Autodesk Fusion 360 part; units mm, degrees
sketch "Sketch2" plane through (0, 0, 0) normal (1, 0, 0) x (0, 0, -1)
  line L0 (0, 0) -> (0, 10)
  dimension "d53" = 10
sketch "Sketch1" plane through (0, 0, 0) normal (0, 1, 0) x (1, 0, 0)
  line L0 (0, 0) -> (141.9, 0)
  line L1 (141.9, 0) -> (141.9, 151.05)
  line L2 (0, 151.05) -> (0, 0)
  line L3 (130.925, 43.6) -> (10.975, 43.6) construction
  circle A0 centre (10.975, 43.6) radius 1.75
  circle A1 centre (130.925, 43.6) radius 1.75
  line L4 (70.95, 0) -> (70.95, 43.6) construction
  line L5 (65.95, 0) -> (68.5, 0)
  line L6 (70.95, -2) -> (65.95, -2)
  line L7 (65.95, -2) -> (65.95, 0)
  line L8 (75.95, -2) -> (75.95, 0)
  line L9 (70.95, -2) -> (75.95, -2)
  line L10 (70.95, 43.6) -> (70.95, 85.6) construction
  line L11 (72.7, 88.1) -> (72.7, 83.1)
  line L12 (69.2, 83.1) -> (69.2, 88.1)
  arc A2 (72.7, 88.1) -> (69.2, 88.1) centre (70.95, 88.1) ccw
  arc A3 (69.2, 83.1) -> (72.7, 83.1) centre (70.95, 83.1) ccw
  line L13 (69.2, 85.6) -> (72.7, 85.6) construction
  line L14 (3.35, 120.45) -> (44.05, 120.45) construction
  circle A4 centre (3.35, 120.45) radius 1.75
  circle A5 centre (44.05, 120.45) radius 1.75
  line L15 (23.7, 151.05) -> (23.7, 120.45) construction
  line L16 (7.7, 149.45) -> (39.7, 149.45)
  line L17 (39.7, 149.45) -> (39.7, 91.45)
  line L18 (39.7, 91.45) -> (7.7, 91.45)
  line L19 (7.7, 91.45) -> (7.7, 149.45)
  line L20 (134.2, 91.45) -> (134.2, 149.45)
  line L21 (134.2, 149.45) -> (102.2, 149.45)
  line L22 (102.2, 149.45) -> (102.2, 91.45)
  circle A6 centre (138.55, 120.45) radius 1.75
  line L23 (102.2, 91.45) -> (134.2, 91.45)
  circle A7 centre (97.85, 120.45) radius 1.75
  line L24 (48.95, 135.45) -> (92.95, 135.45)
  line L25 (92.95, 135.45) -> (92.95, 91.45)
  line L26 (92.95, 91.45) -> (48.95, 91.45)
  line L27 (48.95, 91.45) -> (48.95, 135.45)
  line L28 (48.95, 113.45) -> (39.7, 113.45) construction
  line L29 (92.95, 113.45) -> (102.2, 113.45) construction
  circle A8 centre (52.7, 131.7) radius 1.75
  circle A9 centre (52.7, 95.2) radius 1.75
  circle A10 centre (89.2, 95.2) radius 1.75
  circle A11 centre (89.2, 131.7) radius 1.75
  line L30 (74.1, 142.05) -> (74.1, 137.05)
  line L31 (74.1, 173.25) -> (74.1, 168.25)
  line L32 (82.45, 143.65) -> (82.45, 166.65)
  line L33 (74.1, 173.25) -> (79.95, 173.25)
  line L34 (57.85, 142.05) -> (74.1, 142.05)
  line L35 (74.1, 168.25) -> (57.85, 168.25)
  line L36 (57.85, 142.05) -> (57.85, 168.25)
  line L37 (78.35, 138.65) -> (78.35, 143.65)
  line L38 (78.35, 166.65) -> (78.35, 171.65)
  line L39 (82.45, 166.65) -> (78.35, 166.65)
  line L40 (78.35, 143.65) -> (82.45, 143.65)
  line L41 (75.7, 166.65) -> (59.45, 166.65)
  line L42 (59.45, 166.65) -> (59.45, 143.65)
  line L43 (75.7, 171.65) -> (75.7, 166.65)
  line L44 (59.45, 143.65) -> (75.7, 143.65)
  line L45 (78.35, 171.65) -> (75.7, 171.65)
  line L46 (75.7, 138.65) -> (78.35, 138.65)
  line L47 (75.7, 143.65) -> (75.7, 138.65)
  line L48 (84.05, 142.05) -> (79.95, 142.05)
  line L49 (79.95, 137.05) -> (74.1, 137.05)
  line L50 (84.05, 168.25) -> (84.05, 142.05)
  line L51 (79.95, 142.05) -> (79.95, 137.05)
  line L52 (79.95, 168.25) -> (79.95, 173.25)
  line L53 (84.05, 168.25) -> (79.95, 168.25)
  line L54 (82.45, 155.15) -> (59.45, 155.15) construction
  line L55 (70.95, 155.15) -> (70.95, 135.45) construction
  line L56 (56.25, 151.05) -> (56.25, 174.85)
  line L57 (56.25, 174.85) -> (85.65, 174.85)
  line L58 (85.65, 174.85) -> (85.65, 151.05)
  line L59 (141.9, 151.05) -> (85.65, 151.05)
  line L60 (56.25, 151.05) -> (0, 151.05)
  line L61 (59.45, 143.65) -> (57.85, 143.65)
  line L62 (59.45, 147.65) -> (57.85, 147.65)
  line L63 (74.1, 173.25) -> (57.85, 173.25)
  line L64 (57.85, 173.25) -> (57.85, 168.25)
  line L65 (79.95, 173.25) -> (84.05, 173.25)
  line L66 (84.05, 173.25) -> (84.05, 168.25)
  line L67 (75.95, -2) -> (75.95, -3.6)
  line L68 (75.95, -3.6) -> (65.95, -3.6)
  line L69 (65.95, -3.6) -> (65.95, -2)
  point P0 (70.95, 113.45)
  point P1 (-289, 70)
  dimension "d1" = 141.9
  dimension "d2" = 151.05
  dimension "d3" = 119.95
  dimension "d4" = 3.5
  dimension "d6" = 5
  dimension "d8" = 43.6
  dimension "d9" = 42
  dimension "d10" = 3.5
  dimension "d11" = 5
  dimension "d12" = 40.7
  dimension "d13" = 3.5
  dimension "d14" = 3.35
  dimension "d15" = 30.6
  dimension "d16" = 58
  dimension "d17" = 1.6
  dimension "d18" = 32
  dimension "d19" = 16
  dimension "d20" = 44
  dimension "d23" = 44
  dimension "d24" = 3.35
  dimension "d25" = 3.5
  dimension "d26" = 3.75
  dimension "d27" = 3.75
  dimension "d28" = 22
  dimension "d29" = 22
  dimension "d31" = 360
  dimension "d32" = 4.9
  dimension "d33" = 4.9
  dimension "d34" = 1.6
  dimension "d35" = 1.6
  dimension "d36" = 1.6
  dimension "d37" = 1.6
  dimension "d38" = 1.6
  dimension "d39" = 1.6
  dimension "d40" = 1.6
  dimension "d41" = 1.6
  dimension "d42" = 1.6
  dimension "d43" = 1.6
  dimension "d44" = 1.6
  dimension "d45" = 1.6
  dimension "d47" = 5
  dimension "d48" = 23
  dimension "d49" = 23
  dimension "d50" = 4.1
  dimension "d51" = 6.75
  dimension "d54" = 1.6
  dimension "d55" = 1.6
  dimension "d56" = 1.6
  dimension "d57" = 1.6
  dimension "d58" = 4
  dimension "d80" = 2
  dimension "d81" = 1.6
extrude "Extrude1" add sketch "Sketch1" against normal blind 4 contours L0 L1 L2 L5 L56 L57 L58 L59 L60 | L0 L5 L6 L7 L8 L9 | L6 L9 L67 L68 L69 | L16 L17 L18 L19 | L20 L21 L22 L23 | L24 L25 L26 L27 | L30 L31 L32 L33 L34 L35 L36 L37 L38 L39 L40 L41 L42 L43 L44 L45 L46 L47 L48 L49 L50 L51 L52 L53 L61 L62 | L36 L42 L61 L62 | L32 L37 L38 L39 L40 L41 L42 L43 L44 L45 L46 L47 | L31 L35 L63 L64 | L52 L53 L65 L66
extrude "Extrude2" cut sketch "Sketch1" against normal blind 1.6 contours L16 L17 L18 L19 | L20 L21 L22 L23 | L24 L25 L26 L27
extrude "Extrude3" add sketch "Sketch1" along normal blind 5 contours L6 L9 L67 L68 L69
extrude "Extrude4" add sketch "Sketch1" along normal blind 40 contours L30 L31 L32 L33 L34 L35 L36 L37 L38 L39 L40 L41 L42 L43 L44 L45 L46 L47 L48 L49 L50 L51 L52 L53 L61 L62 | L31 L35 L63 L64 | L52 L53 L65 L66
sketch "Sketch3" plane through (84.05, 0, 0) normal (1, 0, 0) x (0, 0, -1)
  line L0 (142.05, 0) -> (173.25, 0)
  line L1 (173.25, 0) -> (173.25, 40)
  line L2 (173.25, 40) -> (142.05, 40)
  line L3 (142.05, 40) -> (142.05, 0)
  line L4 (143.65, 0) -> (143.65, 40)
  line L5 (155.65, 43) -> (154.8462, 43)
  line L6 (155.65, 37) -> (154.8462, 37)
  arc A0 (155.65, 37) -> (155.65, 43) centre (155.65, 40) ccw
  arc A1 (154.8462, 43) -> (154.8462, 37) centre (149.65, 40) ccw
  dimension "d69" = 6
  dimension "d70" = 12
  dimension "d71" = 6
extrude "Extrude6" cut sketch "Sketch3" against normal blind 5 contours L2 L6 A0 A1
ref_plane "WorkPlane1" through (66.775, 20, -157.65) normal (0, 0, -1) x (-1, 0, 0)
sketch "Sketch4" plane through (66.775, 20, -157.65) normal (0, 0, -1) x (1, 0, 0)
  line L0 (-7.325, 20) -> (-7.325, -20)
  line L1 (-7.325, -20) -> (-7.325, 20)
  line L2 (-7.325, -5.5787) -> (-7.325, -0.4998)
  line L3 (8.925, 20) -> (-7.325, 20)
  line L4 (-7.325, -5.5787) -> (7.1393, 20)
  line L5 (-7.325, -0.4998) -> (4.2673, 20)
  line L6 (4.2673, 20) -> (7.1393, 20)
  dimension "d77" = 2.5
extrude "Extrude7" add sketch "Sketch4" along normal mid plane 1.6 contours L0 L1 L2 L3 L4 L5 L6
equation "d15 = ( 58 / 2 ) * 1 mm + 1.6 mm"
equation "d34 = d44"
equation "d35 = d44"
equation "d36 = d44"
equation "d37 = d44"
equation "d38 = d44"
equation "d39 = d44"
equation "d40 = d44"
equation "d41 = d44"
equation "d42 = d44"
equation "d43 = d44"
equation "d45 = d44"
equation "d56 = d34"
equation "d57 = d55"
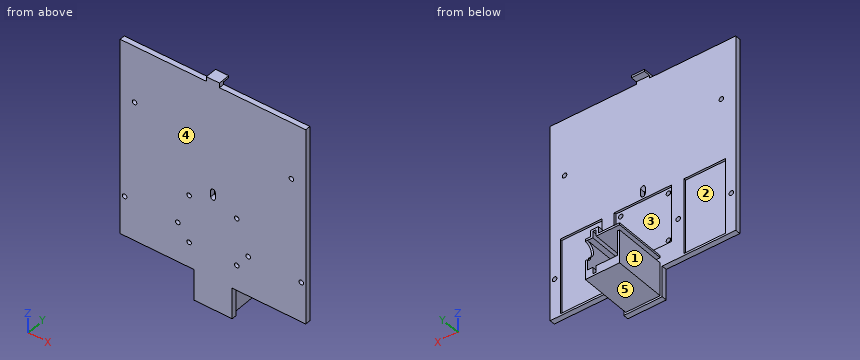
Work out the finished part from the listing and answer in its coordinate system (mm). Face numbers are marked on the shaded views. A direction names the side the tool comes from. Round coordinates to 2 decimals unless told otherwise and drop trailing zeros. Write each loop counter-clockwise with the first axis right and the second up, starting at its lowest first coordinate (ties: lowest second). Pieces come first, ordered by that corner, then holes. Notation, with made-up numbers: (88.5, 89) -> (122.5, 89) arc R38 cw to (122.5, 128) -> close; hole circle Ø6 at (-25.5, -18.5). An arc over 180 degrees is marked (long way). Answer as CSV lines item,"result". Start each with the question number.
(1) The part is cut by section A-A, the plane x = 119. Give the vertices of the cut face in (y, z), then the cut area to 3 significant figures.
(2) A tool of negligible diameter and unlimited length cuts with its end or side. For the marked faces 1 and 2, from which of +Z, -Z, +X, -X, +Y, -Y can it reach the whole face along a straight path? Write none if from no direction.
(3) The part is cut by section C-C, the plane z = -38. Give the vertices of the cut face in (x, y), then the cut area to 3 significant figures.
(4) The mould has two halves that part along Z. Classify the marked faces 3, 4 and 5: +Z half, -Z half, draft (parallel to the pull), parting line (faces both ways), or undercut.
(5) Find the intervals of material crossed by probe 1 along X at (y, z) = (-2.3, -95.2); probe 2 along Z at (x, y) = (70, 3.5); probe 3 along X at (y, z) = (30, -160), in increasing order.
(6) Each of these flat-tipped pins is pushed along its axis until it touches: pin 1 (0.5 mm diameter, centred on x = 79, y = -1, fed in from +Z); pin 2 (3 mm diameter, centred on x = 113, y = -2, fed in from -Z); pin 3 (5 mm diameter, centred on x = 82, y = 19, fed in from +Z); pin 4 (2 mm diameter, centred on x = 52.7, z = -95.2, fed in from -Y). Where does it stop, or does it pass through?
(7) The part is cut by section B-B, the plane y = 14.5. Give the vertices of the cut face in (x, z).
Output values:
1,outline,"(-4, -151.05) -> (0, -151.05) -> (0, -149.45) -> (-1.6, -149.45) -> (-1.6, -91.45) -> (0, -91.45) -> (0, 0) -> (-4, 0) -> close"
1,area,"511 mm²"
2,face 1,"+Z, -Z, -X, +Y"
2,face 2,"+Y"
3,outline,"(0, -4) -> (141.9, -4) -> (141.9, 0) -> (0, 0) -> close"
3,area,"568 mm²"
4,face 3,"undercut"
4,face 4,"draft"
4,face 5,"-Z half"
5,probe 1,"x = 0 to 50.95, 54.45 to 87.45, 90.95 to 141.9"
5,probe 2,"z = -173.25 to -166.65, -158.45 to -156.85, -143.65 to -142.05, 2 to 3.6"
5,probe 3,"x = 57.85 to 59.45, 82.45 to 84.05"
6,pin 1,"stops at z = 0"
6,pin 2,"stops at z = -151.05"
6,pin 3,"stops at z = -137.05"
6,pin 4,"passes through"
7,outline,"(57.85, -173.25) -> (84.05, -173.25) -> (84.05, -142.05) -> (79.95, -142.05) -> (79.95, -137.05) -> (74.1, -137.05) -> (74.1, -142.05) -> (57.85, -142.05) -> (57.85, -143.65) -> (75.7, -143.65) -> (75.7, -138.65) -> (78.35, -138.65) -> (78.35, -143.65) -> (82.45, -143.65) -> (82.45, -166.65) -> (78.35, -166.65) -> (78.35, -171.65) -> (75.7, -171.65) -> (75.7, -166.65) -> (59.45, -166.65) -> (59.45, -147.65) -> (57.85, -147.65) -> close; (62.84, -158.45) -> (65.71, -158.45) -> (65.71, -156.85) -> (62.84, -156.85) -> close"
